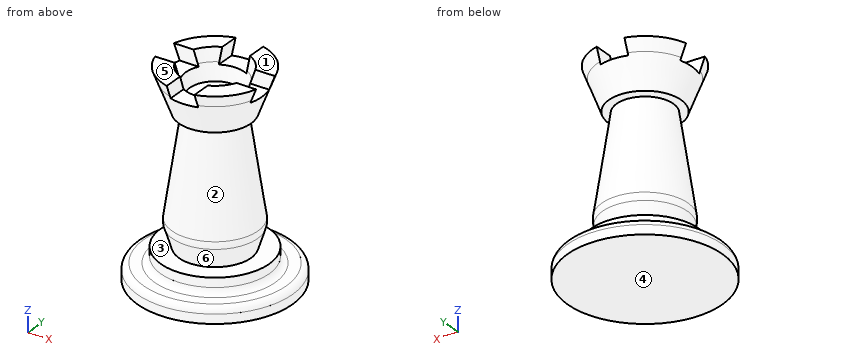
```python
from build123d import *

# Parameters (mm, degrees)
F0_R          = 12.7
F0_R_2        = 8.89
F0_R_3        = 6.35
F0_R_4        = 3.81
F1_DEPTH      = 2.54
F2_DEPTH      = 2.54
F3_R          = 1.016
F7_DEPTH      = 25.4
F7_DEPTH_BACK = 25.4
F9_DEPTH      = 25.4
F9_DEPTH_BACK = 25.4


with BuildPart() as f1:
    # F0 (on Top) → F1 (new body)
    with BuildSketch(Plane.XY):
        Circle(F0_R)
        Circle(F0_R_2, mode=Mode.SUBTRACT)
        Circle(F0_R_2)
        Circle(F0_R_3, mode=Mode.SUBTRACT)
        Circle(F0_R_3)
        Circle(F0_R_4, mode=Mode.SUBTRACT)
        Circle(F0_R_4)
    extrude(amount=-F1_DEPTH)

    # F0 (on Top) → F2 (join)
    with BuildSketch(Plane.XY):
        Circle(F0_R_2)
        Circle(F0_R_3, mode=Mode.SUBTRACT)
        Circle(F0_R_3)
        Circle(F0_R_4, mode=Mode.SUBTRACT)
        Circle(F0_R_4)
    extrude(amount=F2_DEPTH)

    # F3
    f3_edges = [f1.edges().sort_by_distance(p)[0] for p in [
        (-8.89, 0, 0),
        (-12.7, 0, 0),
    ]]
    fillet(f3_edges, radius=F3_R)

    # F4 (on Right) → F5 (revolve)
    with BuildSketch(Plane.YZ):
        with BuildLine():
            ThreePointArc((-7.052727852, 7.0721389887), (-7.0740632783, 6.4527327622), (-6.95464605, 5.8445725864))
            Line((-6.95464605, 5.8445725864), (-5.8483541943, 2.3676548153))
            Line((-5.8483541943, 2.3676548153), (0, 2.3676548153))
            Line((0, 2.3676548153), (0, 21.9140928239))
            Line((0, 21.9140928239), (0, 23.5729362753))
            Line((0, 23.5729362753), (0, 24.7111208737))
            Line((0, 24.7111208737), (0, 24.8141754419))
            Line((0, 24.8141754419), (0, 25.781949982))
            Line((0, 25.781949982), (-4.1019017808, 25.781949982))
            Line((-4.1019017808, 25.781949982), (-4.9252421595, 28.3628571779))
            Line((-4.9252421595, 28.3628571779), (-5.5563063145, 30.341040273))
            Line((-5.5563063145, 30.341040273), (-5.6435932728, 30.341040273))
            Line((-5.6435932728, 30.341040273), (-8.5902156056, 30.341040273))
            Line((-8.5902156056, 30.341040273), (-7.8381793573, 28.3628571779))
            Line((-7.8381793573, 28.3628571779), (-5.9250046527, 23.33037388))
            Line((-5.9250046527, 23.33037388), (-4.647559738, 23.1391453645))
            Line((-4.647559738, 23.1391453645), (-7.052727852, 7.0721389887))
        make_face()
    revolve(axis=Axis((0, 0, 13.5393878445), (0, 0, -1)))

    # F6 (on Front) → F7 (cut, two sides)
    with BuildSketch(Plane.XZ) as f7_sk:
        Polygon((-2.2698096, 28.0051901937), (0, 28.0051901937), (2.2698096, 28.0051901937), (2.2698096, 30.4731242359), (0, 30.4731242359), (-2.2698096, 30.4731242359), align=None)
    extrude(amount=-F7_DEPTH, mode=Mode.SUBTRACT)
    extrude(f7_sk.sketch, amount=F7_DEPTH_BACK, mode=Mode.SUBTRACT)

    # F8 (on Right) → F9 (cut, two sides)
    with BuildSketch(Plane.YZ) as f9_sk:
        Polygon((-2.2698075, 27.955027986), (0, 27.955027986), (2.2698075, 27.955027986), (2.2698075, 31.4495795649), (0, 31.4495795649), (-2.2698075, 31.4495795649), align=None)
    extrude(amount=-F9_DEPTH, mode=Mode.SUBTRACT)
    extrude(f9_sk.sketch, amount=F9_DEPTH_BACK, mode=Mode.SUBTRACT)


solid = f1.part
```
For this review, take the finished solid that the model builds, in its own axes (mm). Face numbers are marked on the shaded views. A direction names the side the tool comes from. Coordinates: 2 decimals unless noted, no trailing zeros. Write each loop counter-clockwise with the first axis right and the second up, starting at its lowest first coordinate (ties: lowest second). Pieces come first, ordered by that corner, then holes. Notation, with made-up numbers: (10, 3.25) - (39, 3.25) arc R25 cw to (39, 35.25) - close; hole circle Ø5 at (26, 26). An arc over 180 degrees is marked (long way). Answer in a Markdown table with one row per item. Add a question column.
Q1. We need section C-C, the plane z = 17. State the section outline as (x, y) points, and give its area (3 significant figures).
Q2. For P1, Ø4, axis at y = -6.5, z = 12.5, coming from the -X side; P2, Ø1.9, axis at x = -6, z = 29, coming from the +Y side; P3, Ø8, axis at y = 5.5, z = 21.5, coming from the +X side; P4, Ø5, axis at y = -10, z = 13.5, coming from the -X side, all flat-tipped, find the tip position at first contact; note any pin that passes through.
Q3. We need section A-A, the plane y = 0. State the section outline as (x, z) points (3 decimals), and give its area (3 significant figures).
Q4. For probe 1 along Z at (x, y) = (-7.75, -0.5); probe 2 along Z at (x, y) = (-0.5, 2.5); probe 3 along Y at (x, z) = (-2.75, 4.5), list the stretches that pass through material, from the lowest coordinate up.
Q5. Tool access review of the marked faces 1 and 2: name each direction out of +Z, -Z, +X, -X, +Y, -Y from which nothing blocks a thin tool from reaching the whole face with its end or side.
Q6. Draft analysis for pull direction Z (two halves, no side actions). For the marked faces 3, 4, 5 and 6, state which applies: +Z half, -Z half, draft (parallel to the pull), parting line (faces both ways), or undercut.
Q7. We need section B-B, the plane x = 0. State the section outline as (y, z) points (3 decimals), and give its area (3 significant figures).
Q8. We need section D-D, the plane z = 12. State the section outline as (x, y) points, and give its area (3 significant figures).
Answer list:
| question | item | result |
|---|---|---|
| 1 | outline | circle Ø11.13 at (0, 0) |
| 1 | area | 97.3 mm2 |
| 2 | P1 | stops at x = -4.37 |
| 2 | P2 | stops at y = 6.44 |
| 2 | P3 | stops at x = 5.71 |
| 2 | P4 | passes through |
| 3 | outline | (-12.7, -2.54) - (12.7, -2.54) - (12.7, -1.016) arc R1.016 ccw to (11.684, 0) - (9.906, 0) arc R1.016 cw to (8.89, 1.016) - (8.89, 2.54) - (5.903, 2.54) - (6.955, 5.845) arc R2.72 ccw to (7.053, 7.072) - (4.648, 23.139) - (5.925, 23.33) - (7.683, 27.955) - (4.795, 27.955) - (4.102, 25.782) - (-4.102, 25.782) - (-4.795, 27.955) - (-7.683, 27.955) - (-5.925, 23.33) - (-4.648, 23.139) - (-7.053, 7.072) arc R2.72 ccw to (-6.955, 5.845) - (-5.903, 2.54) - (-8.89, 2.54) - (-8.89, 1.016) arc R1.016 cw to (-9.906, 0) - (-11.684, 0) arc R1.016 ccw to (-12.7, -1.016) - close |
| 3 | area | 403 mm2 |
| 4 | probe 1 | z = -2.54 to 2.54 |
| 4 | probe 2 | z = -2.54 to 25.78 |
| 4 | probe 3 | y = -5.92 to 5.92 |
| 5 | face 1 | +Z, +X, -X, +Y, -Y |
| 5 | face 2 | none |
| 6 | face 3 | undercut |
| 6 | face 4 | -Z half |
| 6 | face 5 | +Z half |
| 6 | face 6 | undercut |
| 7 | outline | (-12.7, -2.54) - (12.7, -2.54) - (12.7, -1.016) arc R1.016 ccw to (11.684, 0) - (9.906, 0) arc R1.016 cw to (8.89, 1.016) - (8.89, 2.54) - (5.903, 2.54) - (6.955, 5.845) arc R2.72 ccw to (7.053, 7.072) - (4.648, 23.139) - (5.925, 23.33) - (7.702, 28.005) - (4.811, 28.005) - (4.102, 25.782) - (-4.102, 25.782) - (-4.811, 28.005) - (-7.702, 28.005) - (-5.925, 23.33) - (-4.648, 23.139) - (-7.053, 7.072) arc R2.72 ccw to (-6.955, 5.845) - (-5.903, 2.54) - (-8.89, 2.54) - (-8.89, 1.016) arc R1.016 cw to (-9.906, 0) - (-11.684, 0) arc R1.016 ccw to (-12.7, -1.016) - close |
| 7 | area | 403 mm2 |
| 8 | outline | circle Ø12.63 at (0, 0) |
| 8 | area | 125 mm2 |
